Design review of the part built by this model. Coordinates are the model's own, in mm. Face numbers are marked on the shaded views. A direction names the side the tool comes from. Coordinates: 2 decimals unless noted, no trailing zeros. Order: outer loops, then holes, each group sorted by start corner. A loop starts at its lowest first (then second) coordinate and runs counter-clockwise, first axis right, second up. Notation, with made-up numbers: M -23.75,-38 L -14.75,-38 A11 ccw -14.75,-24 Z; hole C 52,-16 d6. An arc over 180 degrees is marked long. Use CSV: the item, a comma, the result in double quotes.
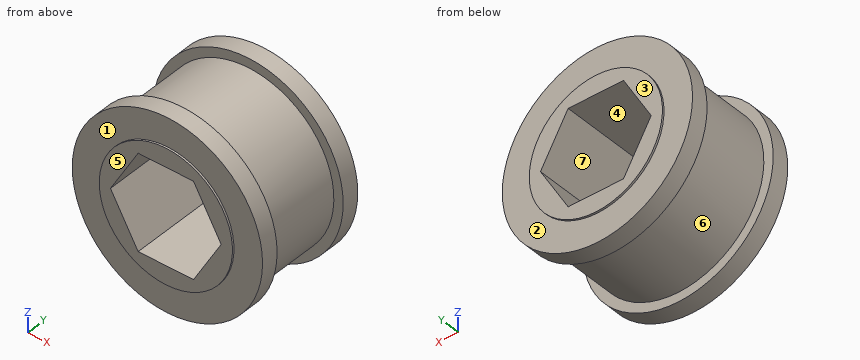
```python
from build123d import *

# Parameters (mm, degrees)
CUT_EXTRUDE1_DEPTH      = 1
CUT_EXTRUDE1_DEPTH_BACK = 16.875


with BuildPart() as part:
    # Sketch2 → Revolve1 (revolve)
    with BuildSketch(Plane(origin=(0, 0, 0), x_dir=(0, 0, -1), z_dir=(1, 0, 0))):
        Polygon((2.54, -3.2131), (8.89, -3.2131), (8.89, -3.4671), (12.7, -3.4671), (12.7, -5.8166), (11.4554, -5.8166), (11.4554, -16.4846), (12.7, -16.4846), (12.7, -18.8341), (8.89, -18.8341), (8.89, -19.0881), (2.54, -19.0881), align=None)
    revolve(axis=Axis((0, 55, 0), (0, -1, 0)))

    # Sketch3 → Cut-Extrude1 (cut, two sides)
    with BuildSketch(Plane(origin=(0, -3.2131, 0), x_dir=(1, 0, 0), z_dir=(0, 1, 0))) as cut_extrude1_sk:
        Polygon((3.695503603, 6.4008), (-3.695503603, 6.4008), (-7.391007206, 0), (-3.695503603, -6.4008), (3.695503603, -6.4008), (7.391007206, 0), align=None)
    extrude(amount=CUT_EXTRUDE1_DEPTH, mode=Mode.SUBTRACT)
    extrude(cut_extrude1_sk.sketch, amount=-CUT_EXTRUDE1_DEPTH_BACK, mode=Mode.SUBTRACT)


solid = part.part
```
(1) Add section A-A on y = -13. State the section outline as (x, z) points, and give its area (3 significant figures).
The answers:
outline,"C 0,0 d22.91; hole M -7.39,0 L -3.7,-6.4 L 3.7,-6.4 L 7.39,0 L 3.7,6.4 L -3.7,6.4 Z"
area,"270 mm2"
(2) Add section D-D on z = 7.5. State the section outline as (x, y) points.
The answers:
outline,"M -10.25,-18.83 L -4.77,-18.83 L -4.77,-19.09 L 4.77,-19.09 L 4.77,-18.83 L 10.25,-18.83 L 10.25,-16.48 L 8.66,-16.48 L 8.66,-5.82 L 10.25,-5.82 L 10.25,-3.47 L 4.77,-3.47 L 4.77,-3.21 L -4.77,-3.21 L -4.77,-3.47 L -10.25,-3.47 L -10.25,-5.82 L -8.66,-5.82 L -8.66,-16.48 L -10.25,-16.48 Z"
(3) The part is to be moulded in two halves that separate along Z. For the marked faces 5, 6 and 7, say which applies: pulls with the +Z half, pulls with the -Z half, needs draft (parallel to the pull), parting line crosses it, or undercut.
The answers:
face 5,"needs draft"
face 6,"parting line crosses it"
face 7,"undercut"
(4) Add section B-B on z = 4.25. State the section outline as (x, y) points, and give its area (3 significant figures).
The answers:
outline,"M -11.97,-18.83 L -7.81,-18.83 L -7.81,-19.09 L -4.94,-19.09 L -4.94,-3.21 L -7.81,-3.21 L -7.81,-3.47 L -11.97,-3.47 L -11.97,-5.82 L -10.64,-5.82 L -10.64,-16.48 L -11.97,-16.48 Z; M 4.94,-19.09 L 7.81,-19.09 L 7.81,-18.83 L 11.97,-18.83 L 11.97,-16.48 L 10.64,-16.48 L 10.64,-5.82 L 11.97,-5.82 L 11.97,-3.47 L 7.81,-3.47 L 7.81,-3.21 L 4.94,-3.21 Z"
area,"191 mm2"
(5) Clearance check with flat-ended pins moving along their axes: P1, Ø1, axis at x = -0.5, y = -15, coming from the -Z side; P2, Ø8, axis at y = -14.5, z = -6, coming from the -X side; P3, Ø5, axis at x = -8.5, y = -15, coming from the -Z side. State where each tip first meets the part, or that it passes through.
The answers:
P1,"stops at z = -11.46"
P2,"stops at x = -12.45"
P3,"stops at z = -10.92"
(6) Wall thickness on probe 1 along Z at (x, y) = (-0.25, -8.75); probe 2 along Y at (x, z) = (10.75, 1.75); probe 3 along Y at (x, z) = (11.5, 3.5): over which ranges is each line inside the solid? List them lowest first.
The answers:
probe 1,"z = -11.45 to -6.4, 6.4 to 11.45"
probe 2,"y = -18.83 to -3.47"
probe 3,"y = -18.83 to -16.48, -5.82 to -3.47"
(7) Add section C-C on x = 0. State the section outline as (y, z) points, and give its area (3 significant figures).
The answers:
outline,"M -19.09,-8.89 L -18.83,-8.89 L -18.83,-12.7 L -16.48,-12.7 L -16.48,-11.46 L -5.82,-11.46 L -5.82,-12.7 L -3.47,-12.7 L -3.47,-8.89 L -3.21,-8.89 L -3.21,-6.4 L -19.09,-6.4 Z; M -19.09,6.4 L -3.21,6.4 L -3.21,8.89 L -3.47,8.89 L -3.47,12.7 L -5.82,12.7 L -5.82,11.46 L -16.48,11.46 L -16.48,12.7 L -18.83,12.7 L -18.83,8.89 L -19.09,8.89 Z"
area,"170 mm2"
(8) For the marked faces 1, 2, 3 and 4, list the 3-axis set-ups (+Z, -Z, +X, -X, +Y, -Y) from which the entire face can be reached by the end or side of a thin tool; tool diameter is ignored.
The answers:
face 1,"-Y"
face 2,"+Y"
face 3,"+Z, -Z, +X, -X, +Y"
face 4,"+Y, -Y"
